from build123d import *

# Parameters (mm, degrees)
BOSS_EXTRUDE1_DEPTH          = 5.5
SKETCH4_W                    = 16
SKETCH4_H                    = 62.5
SKETCH4_H_2                  = 18
CUT_EXTRUDE1_DEPTH           = 5
SKETCH5_W                    = 18.5
SKETCH5_H                    = 18
CUT_EXTRUDE2_DEPTH           = 3
SKETCH7_W                    = 18
SKETCH7_H                    = 62.5
CUT_EXTRUDE3_DEPTH           = 1.8
CUT_EXTRUDE4_START           = -1
SKETCH10_W                   = 8
SKETCH10_H                   = 1
CUT_EXTRUDE4_DEPTH           = 89.479047827
CUT_EXTRUDE4_TAPER           = -45
CUT_EXTRUDE4_OTHER_WAY_DEPTH = 1.8
FILLET1_R                    = 4
CHAMFER1_SIZE                = 0.5
CHAMFER1_SIZE2               = 0.866025404
CUT_EXTRUDE5_REACH           = 68.817
FILLET2_R                    = 2
FILLET3_R                    = 2


with BuildPart() as part:
    # Sketch2 → Boss-Extrude1 (new body)
    with BuildSketch(Plane.XY):
        with BuildLine():
            Line((-9, 75.5), (9, 75.5))
            ThreePointArc((9, 75.5), (11.121320344, 74.621320344), (12, 72.5))
            Line((12, 72.5), (12, -13))
            ThreePointArc((12, -13), (11.121320344, -15.121320344), (9, -16))
            Line((9, -16), (-9, -16))
            ThreePointArc((-9, -16), (-11.121320344, -15.121320344), (-12, -13))
            Line((-12, -13), (-12, 72.5))
            ThreePointArc((-12, 72.5), (-11.121320344, 74.621320344), (-9, 75.5))
        make_face()
    extrude(amount=BOSS_EXTRUDE1_DEPTH)

    # Sketch4 → Cut-Extrude1 (cut)
    with BuildSketch(Plane.XY.offset(5.5)):
        with Locations((0, 41.25)):
            Rectangle(SKETCH4_W, SKETCH4_H)
        with Locations((0, -4)):
            Rectangle(SKETCH4_W, SKETCH4_H_2)
    extrude(amount=-CUT_EXTRUDE1_DEPTH, mode=Mode.SUBTRACT)

    # Sketch5 → Cut-Extrude2 (cut)
    with BuildSketch(Plane.XY.offset(5.5)):
        with Locations((0, -4)):
            Rectangle(SKETCH5_W, SKETCH5_H)
    extrude(amount=-CUT_EXTRUDE2_DEPTH, mode=Mode.SUBTRACT)

    # Sketch7 → Cut-Extrude3 (cut)
    with BuildSketch(Plane.XY.offset(5.5)):
        with Locations((0, 41.25)):
            Rectangle(SKETCH7_W, SKETCH7_H)
    extrude(amount=-CUT_EXTRUDE3_DEPTH, mode=Mode.SUBTRACT)

    # Sketch10 → Cut-Extrude4 (cut)
    with BuildSketch(Plane.XZ.offset(-72.5).offset(CUT_EXTRUDE4_START)):
        with Locations((0, 5)):
            Rectangle(SKETCH10_W, SKETCH10_H)
    extrude(amount=-CUT_EXTRUDE4_DEPTH, taper=CUT_EXTRUDE4_TAPER, mode=Mode.SUBTRACT)

    # Sketch10 → Cut-Extrude4 other way (cut)
    with BuildSketch(Plane.XZ.offset(-72.5).offset(CUT_EXTRUDE4_START)):
        with Locations((0, 5)):
            Rectangle(SKETCH10_W, SKETCH10_H)
    extrude(amount=CUT_EXTRUDE4_OTHER_WAY_DEPTH, mode=Mode.SUBTRACT)

    # Fillet1
    # the kernel refuses this fillet: 4 mm, written as the material it adds along each edge
    with BuildSketch(Plane(origin=(0.666666667, 70.166666667, 7.833333333), x_dir=(0.4082482904638629, 0.40824829046386407, 0.8164965809277255), z_dir=(0.5773502691896267, 0.5773502691896242, -0.5773502691896265))) as fillet1_piece_1_section:
        with BuildLine():
            CenterArc((FILLET1_R * 0.57735026919, -FILLET1_R), FILLET1_R, 90, 60)
            Line((-FILLET1_R * 0.288675134595, -FILLET1_R * 0.5), (0, 0))
            Line((0, 0), (FILLET1_R * 0.57735026919, 0))
        make_face()
    fillet1_piece_1 = extrude(amount=15.011106999, mode=Mode.PRIVATE)
    fillet1_piece_1 = split(fillet1_piece_1, bisect_by=Plane(origin=(0.666666667, 75.5, 7.833333333), z_dir=(0, -1, 0)), keep=Keep.TOP, mode=Mode.PRIVATE)
    fillet1_piece_1 = split(fillet1_piece_1, bisect_by=Plane(origin=(4, 70.166666667, 7.833333333), z_dir=(-1, 0, 0)), keep=Keep.TOP, mode=Mode.PRIVATE)
    fillet1_piece_1 = split(fillet1_piece_1, bisect_by=Plane(origin=(0.666666667, 70.166666667, 4.5), z_dir=(0, 0, -1)), keep=Keep.TOP, mode=Mode.PRIVATE)
    add(fillet1_piece_1)
    with BuildSketch(Plane(origin=(0.666666667, 70.166666667, 7.833333333), x_dir=(0.4082482904638629, 0.40824829046386407, 0.8164965809277255), z_dir=(0.5773502691896267, 0.5773502691896242, -0.5773502691896265))) as fillet1_piece_2_section:
        with BuildLine():
            CenterArc((FILLET1_R * 0.57735026919, -FILLET1_R), FILLET1_R, 90, 60)
            Line((-FILLET1_R * 0.288675134595, -FILLET1_R * 0.5), (0, 0))
            Line((0, 0), (FILLET1_R * 0.57735026919, 0))
        make_face()
    fillet1_piece_2 = extrude(amount=15.011106999, mode=Mode.PRIVATE)
    fillet1_piece_2 = split(fillet1_piece_2, bisect_by=Plane(origin=(0.666666667, 75.5, 7.833333333), z_dir=(0, -1, 0)), keep=Keep.TOP, mode=Mode.PRIVATE)
    fillet1_piece_2 = split(fillet1_piece_2, bisect_by=Plane(origin=(0.666666667, 70.166666667, 5.5), z_dir=(0, 0, -1)), keep=Keep.TOP, mode=Mode.PRIVATE)
    fillet1_piece_2 = split(fillet1_piece_2, bisect_by=Plane(origin=(4, 70.166666667, 7.833333333), z_dir=(1, 0, 0)), keep=Keep.TOP, mode=Mode.PRIVATE)
    fillet1_piece_2 = split(fillet1_piece_2, bisect_by=Plane(origin=(0.666666667, 70.166666667, 4.5), z_dir=(0, 0, 1)), keep=Keep.TOP, mode=Mode.PRIVATE)
    add(fillet1_piece_2)
    with BuildSketch(Plane(origin=(0.666666667, 70.166666667, 7.833333333), x_dir=(0.4082482904638629, 0.40824829046386407, 0.8164965809277255), z_dir=(0.5773502691896267, 0.5773502691896242, -0.5773502691896265))) as fillet1_piece_3_section:
        with BuildLine():
            CenterArc((FILLET1_R * 0.57735026919, -FILLET1_R), FILLET1_R, 90, 60)
            Line((-FILLET1_R * 0.288675134595, -FILLET1_R * 0.5), (0, 0))
            Line((0, 0), (FILLET1_R * 0.57735026919, 0))
        make_face()
    fillet1_piece_3 = extrude(amount=15.011106999, mode=Mode.PRIVATE)
    fillet1_piece_3 = split(fillet1_piece_3, bisect_by=Plane(origin=(0.666666667, 75.5, 7.833333333), z_dir=(0, -1, 0)), keep=Keep.TOP, mode=Mode.PRIVATE)
    fillet1_piece_3 = split(fillet1_piece_3, bisect_by=Plane(origin=(4, 70.166666667, 7.833333333), z_dir=(1, 0, 0)), keep=Keep.TOP, mode=Mode.PRIVATE)
    fillet1_piece_3 = split(fillet1_piece_3, bisect_by=Plane(origin=(0.666666667, 70.166666667, 4.5), z_dir=(0, 0, -1)), keep=Keep.TOP, mode=Mode.PRIVATE)
    add(fillet1_piece_3)
    with BuildSketch(Plane(origin=(-0.666666667, 70.166666667, 7.833333333), x_dir=(0.8164965809277253, 0.40824829046386424, -0.4082482904638631), z_dir=(-0.5773502691896267, 0.5773502691896242, -0.5773502691896265))) as fillet1_piece_4_section:
        with BuildLine():
            CenterArc((FILLET1_R * 0.57735026919, -FILLET1_R), FILLET1_R, 90, 60)
            Line((-FILLET1_R * 0.288675134595, -FILLET1_R * 0.5), (0, 0))
            Line((0, 0), (FILLET1_R * 0.57735026919, 0))
        make_face()
    fillet1_piece_4 = extrude(amount=15.011106999, mode=Mode.PRIVATE)
    fillet1_piece_4 = split(fillet1_piece_4, bisect_by=Plane(origin=(-0.666666667, 75.5, 7.833333333), z_dir=(0, -1, 0)), keep=Keep.TOP, mode=Mode.PRIVATE)
    fillet1_piece_4 = split(fillet1_piece_4, bisect_by=Plane(origin=(-0.666666667, 70.166666667, 5.5), z_dir=(0, 0, -1)), keep=Keep.TOP, mode=Mode.PRIVATE)
    fillet1_piece_4 = split(fillet1_piece_4, bisect_by=Plane(origin=(-0.666666667, 70.166666667, 4.5), z_dir=(0, 0, 1)), keep=Keep.TOP, mode=Mode.PRIVATE)
    fillet1_piece_4 = split(fillet1_piece_4, bisect_by=Plane(origin=(-4, 70.166666667, 7.833333333), z_dir=(-1, 0, 0)), keep=Keep.TOP, mode=Mode.PRIVATE)
    add(fillet1_piece_4)
    with BuildSketch(Plane(origin=(-0.666666667, 70.166666667, 7.833333333), x_dir=(0.8164965809277253, 0.40824829046386424, -0.4082482904638631), z_dir=(-0.5773502691896267, 0.5773502691896242, -0.5773502691896265))) as fillet1_piece_5_section:
        with BuildLine():
            CenterArc((FILLET1_R * 0.57735026919, -FILLET1_R), FILLET1_R, 90, 60)
            Line((-FILLET1_R * 0.288675134595, -FILLET1_R * 0.5), (0, 0))
            Line((0, 0), (FILLET1_R * 0.57735026919, 0))
        make_face()
    fillet1_piece_5 = extrude(amount=15.011106999, mode=Mode.PRIVATE)
    fillet1_piece_5 = split(fillet1_piece_5, bisect_by=Plane(origin=(-0.666666667, 75.5, 7.833333333), z_dir=(0, -1, 0)), keep=Keep.TOP, mode=Mode.PRIVATE)
    fillet1_piece_5 = split(fillet1_piece_5, bisect_by=Plane(origin=(-0.666666667, 70.166666667, 4.5), z_dir=(0, 0, -1)), keep=Keep.TOP, mode=Mode.PRIVATE)
    fillet1_piece_5 = split(fillet1_piece_5, bisect_by=Plane(origin=(-4, 70.166666667, 7.833333333), z_dir=(1, 0, 0)), keep=Keep.TOP, mode=Mode.PRIVATE)
    add(fillet1_piece_5)
    with BuildSketch(Plane(origin=(-0.666666667, 70.166666667, 7.833333333), x_dir=(0.8164965809277253, 0.40824829046386424, -0.4082482904638631), z_dir=(-0.5773502691896267, 0.5773502691896242, -0.5773502691896265))) as fillet1_piece_6_section:
        with BuildLine():
            CenterArc((FILLET1_R * 0.57735026919, -FILLET1_R), FILLET1_R, 90, 60)
            Line((-FILLET1_R * 0.288675134595, -FILLET1_R * 0.5), (0, 0))
            Line((0, 0), (FILLET1_R * 0.57735026919, 0))
        make_face()
    fillet1_piece_6 = extrude(amount=15.011106999, mode=Mode.PRIVATE)
    fillet1_piece_6 = split(fillet1_piece_6, bisect_by=Plane(origin=(-0.666666667, 75.5, 7.833333333), z_dir=(0, -1, 0)), keep=Keep.TOP, mode=Mode.PRIVATE)
    fillet1_piece_6 = split(fillet1_piece_6, bisect_by=Plane(origin=(-0.666666667, 70.166666667, 4.5), z_dir=(0, 0, -1)), keep=Keep.TOP, mode=Mode.PRIVATE)
    fillet1_piece_6 = split(fillet1_piece_6, bisect_by=Plane(origin=(-4, 70.166666667, 7.833333333), z_dir=(-1, 0, 0)), keep=Keep.TOP, mode=Mode.PRIVATE)
    add(fillet1_piece_6)

    # Chamfer1
    chamfer1_edges = [part.edges().sort_by_distance(p)[0] for p in [
        (0, -13, 5.5),
        (-9.25, -4, 5.5),
        (9.25, -4, 5.5),
        (-9, 41.25, 5.5),
        (9, 41.25, 5.5),
    ]]
    chamfer1_side = [part.faces().sort_by_distance(p)[0] for p in [
        (-5.551441315, 73.803006174, 5.5),
    ]]
    chamfer(chamfer1_edges, length=CHAMFER1_SIZE, length2=CHAMFER1_SIZE2, reference=chamfer1_side[0])

    # Sketch11 → Cut-Extrude5 (cut, up to next)
    with BuildSketch(Plane(origin=(0, 10, 0), x_dir=(1, 0, 0), z_dir=(0, 1, 0)), mode=Mode.PRIVATE) as cut_extrude5_sk1:
        with BuildLine():
            Line((-7, -5.5), (-7, -0.5))
            Line((-7, -0.5), (-3.169880661, -0.5))
            Line((-3.169880661, -0.5), (-3.169880661, -1.341453537))
            ThreePointArc((-3.169880661, -1.341453537), (-3.322121596, -2.106820401), (-3.755667099, -2.755667099))
            Line((-3.755667099, -2.755667099), (-6.5, -5.5))
            Line((-6.5, -5.5), (-7, -5.5))
        make_face()
    cut_extrude5_tool1 = extrude(cut_extrude5_sk1.sketch, amount=-CUT_EXTRUDE5_REACH, mode=Mode.PRIVATE) & part.part
    add(cut_extrude5_tool1.solids().sort_by_distance((-5.426528, 10, 2.435535))[0], mode=Mode.SUBTRACT)

    # Fillet2
    fillet2_edges = [part.edges().sort_by_distance(p)[0] for p in [
        (-3.169880661, 5, 0.920726768),
        (-3.322121596, 5, 2.106820401),
        (-5.12783355, 5, 4.12783355),
        (-5.12783355, 10, 4.12783355),
        (-3.322121596, 10, 2.106820401),
        (-3.169880661, 10, 0.920726768),
    ]]
    fillet(fillet2_edges, radius=FILLET2_R)

    # Fillet3
    fillet3_edges = [part.edges().sort_by_distance(p)[0] for p in [
        (-7, 10, 3),
        (-7, 5, 3),
    ]]
    fillet(fillet3_edges, radius=FILLET3_R)


solid = part.part
Geometry check sheet. Reference: the model listing, model coordinates, mm. A direction names the side the tool comes from. Give positions to 0.01 mm unless a question says otherwise; leave off trailing zeros. Write each loop counter-clockwise with the first axis right and the second up, starting at its lowest first coordinate (ties: lowest second). Pieces come first, ordered by that corner, then holes. Notation, with made-up numbers: (-28, 81) - (14, 81) arc R20 cw to (14, 103) - close; hole circle Ø10 at (0, -39.5). An arc over 180 degrees is marked (long way). Put each result on its own line as item: value.
1. Set-up check for faces 1 (the flat face through (8, -4, 2)), 2 (the cylindrical face through (-2.6, 9.4, 0.9)), 3 (the cylindrical face through (-3.939, 74.584, 3.863)): record each of +Z, -Z, +X, -X, +Y, -Y from which the full face is reachable in a straight line by a thin tool's end or side.
Ans:
face 1: +Z
face 2: none
face 3: +Z, +Y
2. Draft check along X on faces 4 (the cylindrical face through (-11.1, -15.14, 2.71)), 5 (the flat face through (-8, -4, 2)), 6 (the cylindrical face through (-7.4, 5.8, 3)), 7 (the cylindrical face through (11.1, 74.64, 2.71)). Enter one of: +X half, -X half, draft (parallel to the pull), parting line (faces both ways), or undercut.
Ans:
face 4: -X half
face 5: undercut
face 6: undercut
face 7: +X half
3. Thickness scan on line 1 (Y direction, x = 4.5, z = 1.6); line 2 (X direction, y = 29, z = 1.8); line 3 (Y direction, x = -3.5, z = 3.3). Record the ranges inside material, lowest first.
Ans:
line 1: y = -16 to -13, 5 to 10, 72.5 to 75.5
line 2: x = -12 to -8, 8 to 12
line 3: y = -16 to -13, 5.61 to 9.39, 72.5 to 74.83
4. Go/stop test with flat-tipped pins: pin 1 (0.8 mm diameter, centred on x = 8.5, y = 51.5, fed in from +Z); pin 2 (1 mm diameter, centred on x = 9, y = -3.5, fed in from +Z); pin 3 (1.1 mm diameter, centred on x = -8.5, y = 37, fed in from +Z). Record where each tip stops, or that it passes through.
Ans:
pin 1: stops at z = 3.7
pin 2: stops at z = 5.07
pin 3: stops at z = 4.72
5. Sectioned sample at A-A, the plane y = 35. Enter the section's corners in (x, z), plus the area to 3 significant figures.
Ans:
outline: (-12, 0) - (12, 0) - (12, 5.5) - (9.5, 5.5) - (9, 4.63) - (9, 3.7) - (8, 3.7) - (8, 0.5) - (-8, 0.5) - (-8, 3.7) - (-9, 3.7) - (-9, 4.63) - (-9.5, 5.5) - (-12, 5.5) - close
area: 48.0 mm²
6. Sectioned sample at B-B, the plane y = -10. Enter the section's corners in (x, z), plus the area to 3 significant figures.
Ans:
outline: (-12, 0) - (12, 0) - (12, 5.5) - (9.75, 5.5) - (9.25, 4.63) - (9.25, 2.5) - (8, 2.5) - (8, 0.5) - (-8, 0.5) - (-8, 2.5) - (-9.25, 2.5) - (-9.25, 4.63) - (-9.75, 5.5) - (-12, 5.5) - close
area: 44.1 mm²
